Design review of the part shown in the three views and the two pictorial views. Dimensions are in mm from the part's minimum x, y and z. A direction names the side the tool comes from. Give positions to 0.01 mm unless a question says otherwise; leave off trailing zeros. Order: outer loops, then holes, each group sorted by start corner. A loop starts at its lowest first (then second) coordinate and runs counter-clockwise, first axis right, second up. Notation, with made-up numbers: (-18, 52) -> (-10, 52) arc R24 ccw to (-10, 86) -> close; hole circle Ø4 at (-19.5, 87.25). An arc over 180 degrees is marked (long way). Use one line per item in the form item = value.
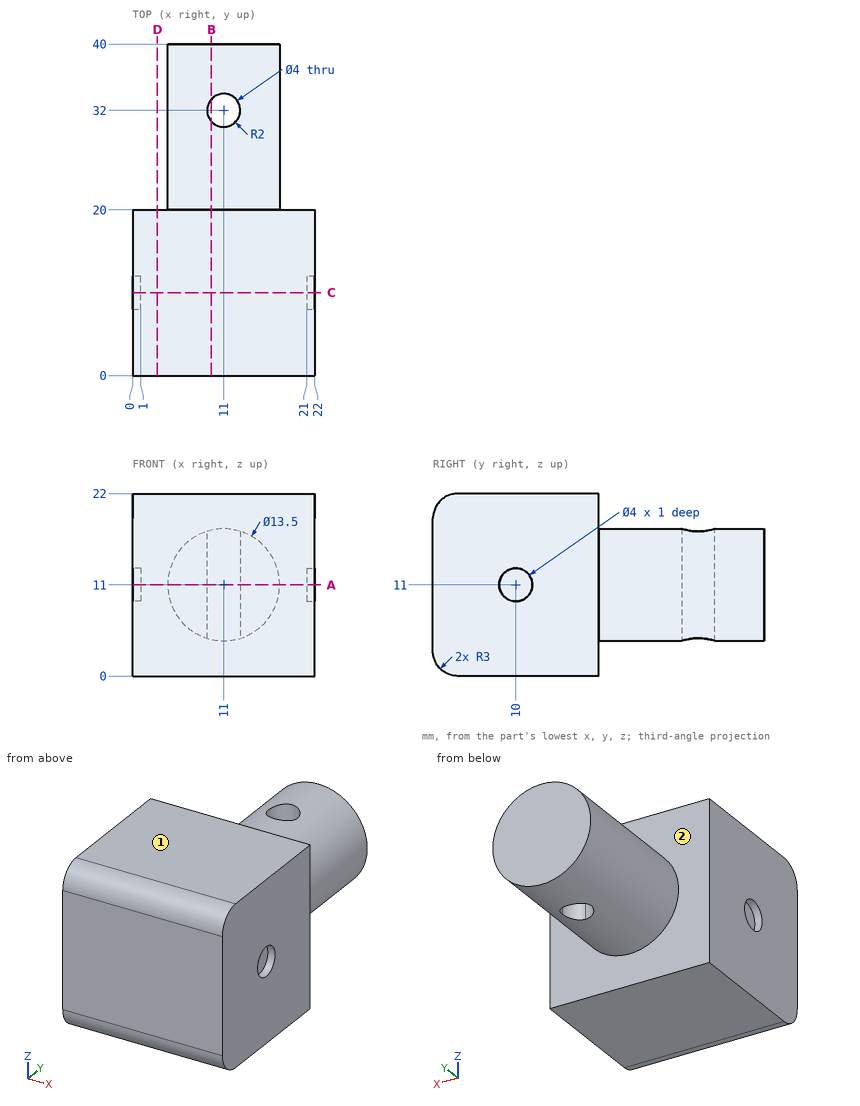
1. Add section A-A on z = 11. Give the boundary of the cut face in (x, y).
Values:
outline = (0, 0) -> (22, 0) -> (22, 8) -> (21, 8) -> (21, 12) -> (22, 12) -> (22, 20) -> (17.75, 20) -> (17.75, 40) -> (4.25, 40) -> (4.25, 20) -> (0, 20) -> (0, 12) -> (1, 12) -> (1, 8) -> (0, 8) -> close; hole (11, 30) arc R2 ccw to (13, 32) arc R2 ccw (long way) to start
2. Add section D-D on x = 3. Give the boundary of the cut face in (y, z).
Values:
outline = (0, 3) arc R3 ccw to (3, 0) -> (20, 0) -> (20, 22) -> (3, 22) arc R3 ccw to (0, 19) -> close
3. For pin 1 Ø1.2 at (y, z) = (10.5, 10) entering from -X; pin 2 Ø2 at (x, y) = (16.5, 30) entering from +Z; pin 3 Ø1 at (y, z) = (28, 2.5) entering from +X; pin 4 Ø6 at (y, z) = (26.5, 9.5) entering from +X, all flat-tipped, find the tip position at first contact; note any pin that passes through.
Values:
pin_1 = 1
pin_2 = 16.03
pin_3 = through
pin_4 = 17.75
4. For L1, parallel to Z at x = 0.5, y = 10; L2, parallel to Y at x = 11, z = 8.75; L3, parallel to Y at x = 2.25, z = 8.5, list the stretches that pass through material, from the lowest coordinate up.
Values:
L1 = 0 to 9, 13 to 22
L2 = 0 to 30, 34 to 40
L3 = 0 to 20
5. Add section C-C on y = 10. Give the boundary of the cut face in (x, z), then the cut area to 3 significant figures.
Values:
outline = (0, 0) -> (22, 0) -> (22, 9) -> (21, 9) -> (21, 13) -> (22, 13) -> (22, 22) -> (0, 22) -> (0, 13) -> (1, 13) -> (1, 9) -> (0, 9) -> close
area = 476 mm^2
6. Add section B-B on x = 9.5. Give the boundary of the cut face in (y, z).
Values:
outline = (0, 3) arc R3 ccw to (3, 0) -> (20, 0) -> (20, 4.42) -> (30.68, 4.42) -> (30.68, 17.58) -> (20, 17.58) -> (20, 22) -> (3, 22) arc R3 ccw to (0, 19) -> close; (33.32, 4.42) -> (40, 4.42) -> (40, 17.58) -> (33.32, 17.58) -> close
7. Tool access review of the marked faces 1 and 2: name each direction out of +Z, -Z, +X, -X, +Y, -Y from which nothing blocks a thin tool from reaching the whole face with its end or side.
Values:
face_1 = +Z, +X, -X, +Y, -Y
face_2 = +Y
